from build123d import *

# Parameters (mm, degrees)
F0_R     = 25.5
F0_R_2   = 24.5
F1_DEPTH = 5
F3_DEPTH = 27.5
F4_R     = 12.5
F5_DEPTH = 30.001


with BuildPart() as f1:
    # F0 (on Front) → F1 (new body)
    with BuildSketch(Plane.XZ):
        with Locations((0, 35.5)):
            Circle(F0_R)
        with Locations((0, 35.5)):
            Circle(F0_R_2, mode=Mode.SUBTRACT)
    extrude(amount=-F1_DEPTH)

    # F2 (on Right) → F3 (join, symmetric)
    with BuildSketch(Plane.YZ):
        Polygon((-30, 0), (0, 0), (0, 65), (-15, 65), align=None)
    extrude(amount=F3_DEPTH, both=True)

    # F4 (on Front) → F5 (cut, through all)
    with BuildSketch(Plane.XZ):
        with BuildLine():
            ThreePointArc((-27.5, 35.5), (0, 63), (27.5, 35.5))
            Line((27.5, 35.5), (32.5, 35.5))
            Line((32.5, 35.5), (32.5, 70))
            Line((32.5, 70), (-32.5, 70))
            Line((-32.5, 70), (-32.5, 35.5))
            Line((-32.5, 35.5), (-27.5, 35.5))
        make_face()
        with Locations((0, 35.5)):
            Circle(F4_R)
    extrude(amount=F5_DEPTH, mode=Mode.SUBTRACT)


solid = f1.part
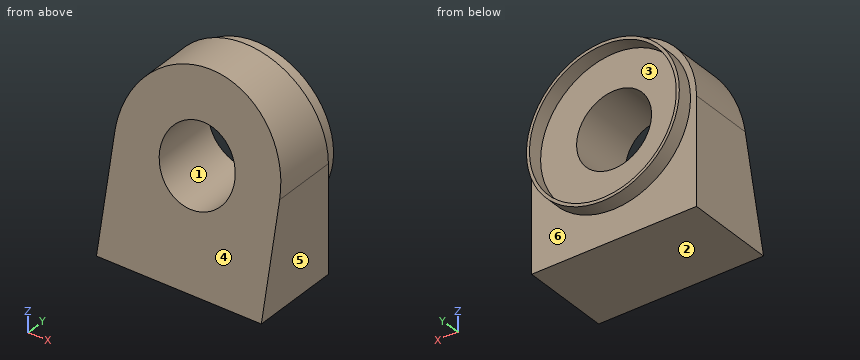
For this review, take the finished solid that the model builds, in its own axes (mm). Face numbers are marked on the shaded views. A direction names the side the tool comes from. Round coordinates to 2 decimals unless told otherwise and drop trailing zeros. Order: outer loops, then holes, each group sorted by start corner. A loop starts at its lowest first (then second) coordinate and runs counter-clockwise, first axis right, second up. Notation, with made-up numbers: M 13,-29.5 L 27,-29.5 A26 ccw 27,-9.5 Z; hole C -32,-38 d11. An arc over 180 degrees is marked long. Use a Markdown table: item, result. Add a question column.
Item 1: Add section A-A, the plane x = -2.5. Give the boundary of the cut face in (y, z), then the cut area to 3 significant figures.
Item 2: To check wall thickness, follow line 1 along Z through (x, y) = (0, 1); line 2 along X through (y, z) = (-13.5, 35.5); line 3 along Z through (x, y) = (0, -19). State the ranges of each line that lie inside material, in increasing order.
Item 3: Add section D-D, the plane z = 16. Give the boundary of the cut face in (x, y), then the cut area to 3 significant figures.
Item 4: Add section B-B, the plane z = 33. Give the boundary of the cut face in (x, y), then the cut area to 3 significant figures.
Item 5: Mouldability with a two-part tool opening along Z and no side actions: class the marked faces 1, 2, 3 and 4 as released by +Z, released by -Z, zero draft, split by the parting line, or undercut.
Item 6: Add section C-C, the plane y = -10.5. Give the boundary of the cut face in (x, z).
Item 7: Tool access review of the marked faces 5 and 6: name each direction out of +Z, -Z, +X, -X, +Y, -Y from which nothing blocks a thin tool from reaching the whole face with its end or side.
Item 8: Insertion check: pin 1 (12 mm diameter, centred on y = -15, z = 54.5, fed in from -X); pin 2 (16.5 mm diameter, centred on x = 4.5, z = 44, fed in from +Y); pin 3 (4 mm diameter, centred on y = -15, z = 47, fed in from +X). Each pin has a flat end and moves straight along its axis. Give the tip position at first contact, or say it passes through.
Geometry results:
| question | item | result |
|---|---|---|
| 1 | outline | M -30,0 L 0,0 L 0,10.12 L 5,10.12 L 5,11.13 L 0,11.13 L 0,23.25 L -24.63,23.25 Z; M -18.98,47.75 L 0,47.75 L 0,59.87 L 5,59.87 L 5,60.88 L 0,60.88 L 0,62.89 L -15.49,62.89 Z |
| 1 | area | 906 mm² |
| 2 | line 1 | z = 10 to 11, 60 to 61 |
| 2 | line 2 | x = -27.5 to -12.5, 12.5 to 27.5 |
| 2 | line 3 | z = 0 to 23 |
| 3 | outline | M -27.5,-26.31 L 27.5,-26.31 L 27.5,0 L 16.43,0 L 16.43,5 L 14.83,5 L 14.83,0 L -14.83,0 L -14.83,5 L -16.43,5 L -16.43,0 L -27.5,0 Z |
| 3 | area | 1,460 mm² |
| 4 | outline | M -27.5,-22.38 L -12.25,-22.38 L -12.25,0 L -24.37,0 L -24.37,5 L -25.38,5 L -25.38,0 L -27.5,0 Z; M 12.25,-22.38 L 27.5,-22.38 L 27.5,0 L 25.38,0 L 25.38,5 L 24.37,5 L 24.37,0 L 12.25,0 Z |
| 4 | area | 693 mm² |
| 5 | face 1 | undercut |
| 5 | face 2 | released by -Z |
| 5 | face 3 | undercut |
| 5 | face 4 | released by +Z |
| 6 | outline | M -27.5,0 L 27.5,0 L 27.5,35.5 A27.5 ccw -27.5,35.5 Z; hole C 0,35.5 d25 |
| 7 | face 5 | +Z, -Z, +X, +Y, -Y |
| 7 | face 6 | +Y |
| 8 | pin 1 | stops at x = -24.23 |
| 8 | pin 2 | stops at y = 0 |
| 8 | pin 3 | stops at x = 25.81 |
